from build123d import *

# Parameters (mm, degrees)
BOSS_EXTRUDE1_DEPTH = 2


with BuildPart() as part:
    # Sketch2 → Boss-Extrude1 (new body)
    with BuildSketch(Plane(origin=(0, 0, 0), x_dir=(1, 0, 0), z_dir=(0, 1, 0))):
        with BuildLine():
            Line((0, 0), (0, 6.63))
            ThreePointArc((0, 6.63), (5.49918056, 3.525064844), (11.346717944, 5.91))
            ThreePointArc((11.346717944, 5.91), (17.433302094, 8.62038484), (23.519886243, 5.91))
            ThreePointArc((23.519886243, 5.91), (28.908302094, 3.510512821), (34.296717944, 5.91))
            ThreePointArc((34.296717944, 5.91), (40.383302094, 8.62038484), (46.469886243, 5.91))
            ThreePointArc((46.469886243, 5.91), (51.858302094, 3.510512821), (57.246717944, 5.91))
            ThreePointArc((57.246717944, 5.91), (63.333302094, 8.62038484), (69.419886243, 5.91))
            Line((69.419886243, 5.91), (69.419886243, 0.34303853))
            ThreePointArc((69.419886243, 0.34303853), (63.282196464, 1.985068989), (57.246717944, 0))
            ThreePointArc((57.246717944, 0), (51.963740367, -1.655479057), (46.680762789, 0))
            ThreePointArc((46.680762789, 0), (40.331907408, 1.989483575), (33.983052027, 0))
            ThreePointArc((33.983052027, 0), (28.915381395, -1.58801026), (23.847710762, 0))
            ThreePointArc((23.847710762, 0), (17.498855381, 1.989483575), (11.15, 0))
            Line((11.15, 0), (0, 0))
        make_face()
    extrude(amount=BOSS_EXTRUDE1_DEPTH)


solid = part.part
Geometry check sheet. Reference: the model listing, model coordinates, mm. A direction names the side the tool comes from. Give positions to 0.01 mm unless a question says otherwise; leave off trailing zeros. Order: outer loops, then holes, each group sorted by start corner. A loop starts at its lowest first (then second) coordinate and runs counter-clockwise, first axis right, second up. Notation, with made-up numbers: (34.5, -2.75) - (80.5, -2.75) arc R22 ccw to (80.5, 35.25) - close; hole circle Ø2 at (38, 71.25). An arc over 180 degrees is marked (long way). Answer as a JSON object with one key per item and string values.
(1) Cross-section at A-A (z = -1). Record the cut outline in (x, y), then the cut area to 3 significant figures.
Report:
{"outline": "(0, 0) - (12.91, 0) - (12.91, 2) - (0, 2) - close; (22.09, 0) - (35.75, 0) - (35.75, 2) - (22.09, 2) - close; (44.92, 0) - (59.01, 0) - (59.01, 2) - (44.92, 2) - close; (68.18, 0) - (69.42, 0) - (69.42, 2) - (68.18, 2) - close", "area": "83.8 mm^2"}
(2) Tool access check on faces 5 (the cylindrical face through (40.43, 0.99, -1.99)), 6 (the flat face through (6, 1, 0)). Record the directions out of +Z, -Z, +X, -X, +Y, -Y that give a thin tool (end or side, any length) a straight path to the whole face; none if there is none.
Report:
{"face 5": "+Z, +Y, -Y", "face 6": "+Z, -X, +Y, -Y"}
(3) Cross-section at D-D (x = 29.5). Record the cut outline in (y, z), then the cut area to 3 significant figures.
Report:
{"outline": "(0, -3.53) - (2, -3.53) - (2, 1.57) - (0, 1.57) - close", "area": "10.2 mm^2"}
(4) Cross-section at B-B (y = 1.1). Record the cut outline in (x, z) (3 decimals).
Report:
{"outline": "(0, -6.63) arc R7.25 cw to (11.347, -5.91) arc R8.189 ccw to (23.52, -5.91) arc R7.25 cw to (34.297, -5.91) arc R8.189 ccw to (46.47, -5.91) arc R7.25 cw to (57.247, -5.91) arc R8.189 ccw to (69.42, -5.91) - (69.42, -0.343) arc R11.125 cw to (57.247, 0) arc R9.257 ccw to (46.681, 0) arc R11.125 cw to (33.983, 0) arc R8.88 ccw to (23.848, 0) arc R11.125 cw to (11.15, 0) - (0, 0) - close"}
(5) Material ranges on line 1 (X direction, y = 1.8, z = -5); line 2 (X direction, y = 1.5, z = -4.75); line 3 (X direction, y = 1.95, z = -8), recorded low to high.
Report:
{"line 1": "0 to 1.56, 10.36 to 24.51, 33.31 to 47.46, 56.26 to 69.42", "line 2": "0 to 1.9, 10.01 to 24.85, 32.96 to 47.8, 55.91 to 69.42", "line 3": "14.31 to 20.56, 37.26 to 43.51, 60.21 to 66.46"}
(6) Draft check along X on faces 1 (the flat face through (0, 1, -3)), 2 (the flat face through (69.42, 1, -3)), 3 (the cylindrical face through (40.29, 0.99, -8.62)), 4 (the flat face through (35, 2, -4)). Enter one of: released by +X, released by -X, zero draft, split by the parting line, or undercut.
Report:
{"face 1": "released by -X", "face 2": "released by +X", "face 3": "undercut", "face 4": "zero draft"}
(7) Cross-section at C-C (x = 16). Record the cut outline in (y, z).
Report:
{"outline": "(0, -8.49) - (2, -8.49) - (2, -1.89) - (0, -1.89) - close"}
